```python
from build123d import *

# Parameters (mm, degrees)
F3_DEPTH = 1.778
F4_R     = 1.4103835631


with BuildPart() as f1:
    # F0 (on Front) → F1 (revolve)
    with BuildSketch(Plane.XZ):
        Polygon((3.175, 5.08), (3.175, 0), (5.715, 0), (6.35, 0.635), (4.191, 5.08), align=None)
    revolve(axis=Axis((0, 0, -0.1242621523), (0, 0, -1)))

    # F2 (on Front) → F3 (join, symmetric)
    with BuildSketch(Plane.XZ):
        with BuildLine():
            Line((-16.9389024071, 11.2239024071), (-6.35, 0.635))
            Line((-6.35, 0.635), (-4.191, 5.08))
            Line((-4.191, 5.08), (-11.088930664, 17.0275663772))
            ThreePointArc((-11.088930664, 17.0275663772), (-14.3112014008, 14.4253913106), (-16.9389024071, 11.2239024071))
        make_face()
        with BuildLine():
            ThreePointArc((16.9389024071, 11.2239024071), (14.3112014008, 14.4253913106), (11.088930664, 17.0275663772))
            Line((11.088930664, 17.0275663772), (4.191, 5.08))
            Line((4.191, 5.08), (6.35, 0.635))
            Line((6.35, 0.635), (16.9389024071, 11.2239024071))
        make_face()
        Polygon((-4.191, 5.08), (-6.35, 0.635), (-5.715, 0), (-3.175, 0), (-3.175, 5.08), align=None)
        Polygon((4.191, 5.08), (3.175, 5.08), (3.175, 0), (5.715, 0), (6.35, 0.635), align=None)
    extrude(amount=F3_DEPTH, both=True)

    # F4 (call 1 of 2: OpenCascade refuses the feature's edges together)
    f4_edges = [f1.edges().sort_by_distance(p)[0] for p in [
        (-7.639965, -1.778, 11.053783),
        (-11.326951, -1.778, 5.611951),
        (-11.326951, 1.778, 5.611951),
        (-7.639965, 1.778, 11.053783),
        (-14.311201, 1.778, 14.425391),
        (-16.938902, 0, 11.223902),
        (-14.311201, -1.778, 14.425391),
        (-11.088931, 0, 17.027566),
    ]]
    fillet(f4_edges, radius=F4_R)

    # F4#2 (call 2 of 2)
    f4_2_edges = [f1.edges().sort_by_distance(p)[0] for p in [
        (11.326951, 1.778, 5.611951),
        (11.326951, -1.778, 5.611951),
        (14.311201, 1.778, 14.425391),
        (11.088931, 0, 17.027566),
        (14.311201, -1.778, 14.425391),
        (16.938902, 0, 11.223902),
        (7.639965, 1.778, 11.053783),
        (7.639965, -1.778, 11.053783),
    ]]
    fillet(f4_2_edges, radius=F4_R)


solid = f1.part
```
Build history of the part. All positions in model axes, mm. A direction names the side the tool comes from. Round coordinates to 2 decimals unless told otherwise and drop trailing zeros. Loops run counter-clockwise (first coordinate to the right, second up) from the corner with the lowest first, then second, coordinate; pieces in that order, holes last.
Item 1: Saw through at A-A (x = 0). List the corners of the cut face in (y, z) (3 decimals).
Item 2: Drill centre lines: line 1 along Z through (x, y) = (4, 0); line 2 along X through (y, z) = (0, 2) (3 decimals); line 3 along Y through (x, z) = (9, 7.5). Where is each one in solid material? Low to high.
Item 3: Two-plate mould, pull along X, no slides. Class faces 6 (the face through (10.69, -1.35, 5.54)), 7 (the face through (7.559, -1.354, 10.109)), 8 (the face through (-10.525, 1.376, 5.41)), 9 (the face through (-0.104, 5.014, 3.383)): released by +X, released by -X, zero draft, split by the parting line, or undercut.
Item 4: Pin check, flat tips, straight feed: P1, Ø4, axis at x = 12, y = -2.5, coming from the +Z side; P2, Ø1, axis at x = 13, z = 12.5, coming from the +Y side; P3, Ø1.5, axis at x = 9, z = 8, coming from the -Y side. Stop position of each tip, or through.
Item 5: Saw through at B-B (y = 0). List the corners of the cut face in (x, z) (3 decimals), then the cut area to 3 significant figures.
Item 6: Which spindle directions (+Z, -Z, +X, -X, +Y, -Y) get a long thin tool onto all of the face, cutting with end or side? Do faces 1 (the face through (7.559, 1.354, 10.109)), 2 (the face through (10, 1.778, 8)), 3 (the face through (-0.69, 3.1, 2.5)), 4 (the face through (-7.64, -1.35, 10.26)), 5 (the face through (7.296, -0.005, 10.458)). Say none if no direction does.
Worked answers:
1. outline: (-6.35, 0.635) - (-5.715, 0) - (-3.175, 0) - (-3.175, 5.08) - (-4.191, 5.08) - close; (3.175, 0) - (5.715, 0) - (6.35, 0.635) - (4.191, 5.08) - (3.175, 5.08) - close
2. line 1: z = 0 to 5.08
2. line 2: x = -7.715 to -3.175, 3.175 to 7.715
2. line 3: y = -1.78 to 1.78
3. face 6: released by +X
3. face 7: undercut
3. face 8: released by -X
3. face 9: split by the parting line
4. P1: stops at z = 16.38
4. P2: stops at y = 1.78
4. P3: stops at y = -1.78
5. outline: (-16.228, 12.23) arc R1.41 ccw to (-16.099, 10.384) - (-5.715, 0) - (-3.175, 0) - (-3.175, 5.08) - (-4.191, 5.08) - (-10.315, 15.688) arc R1.41 ccw to (-12.397, 16.1) arc R20.32 ccw to start; (3.175, 0) - (5.715, 0) - (16.099, 10.384) arc R1.41 ccw to (16.228, 12.23) arc R20.32 ccw to (12.397, 16.1) arc R1.41 ccw to (10.315, 15.688) - (4.191, 5.08) - (3.175, 5.08) - close
5. area: 205 mm2
6. face 1: +Z, +Y
6. face 2: +Z, +X, +Y
6. face 3: +Z, -Z
6. face 4: +Z, -Y
6. face 5: +Z, +Y, -Y
